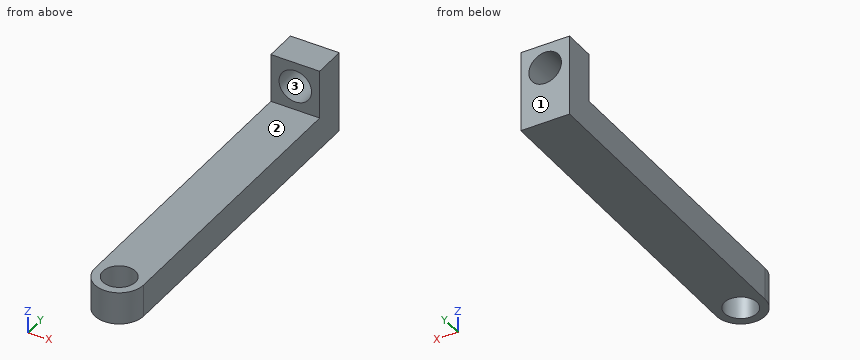
Autodesk Inventor part; units mm, degrees
ref_plane "YZ Plane" through (0, 0, 0) normal (1, 0, 0) x (0, 1, 0)
ref_plane "XZ Plane" through (0, 0, 0) normal (0, 1, 0) x (-1, 0, 0)
ref_plane "XY Plane" through (0, 0, 0) normal (0, 0, 1) x (1, 0, 0)
sketch "草圖1" plane through (0, 0, 0) normal (0, 0, 1) x (1, 0, 0)
  circle A0 centre (0, 0) radius 5
  line L0 (0, 0) -> (0, 100) construction
  line L1 (-7.5, 0) -> (-7.5, 100)
  line L2 (7.5, 100) -> (7.5, 0)
  arc A1 (-7.5, 0) -> (7.5, 0) centre (0, 0) ccw
  arc A2 (7.5, 100) -> (-7.5, 100) centre (0, 100) ccw
  line L3 (-7.5, 100) -> (7.5, 100)
  point P0 (0, 50)
  dimension "d0" = 10
  dimension "d1" = 15
  dimension "d2" = 100
extrude "擠出1" add sketch "草圖1" along normal blind 10 contours L1 L3 L2 A1
sketch "草圖2" plane through (-7.5, 100, 0) normal (0, 1, 0) x (1, 0, 0)
  line L0 (15, -10) -> (0, -10)
  line L1 (15, -25) -> (0, -25)
  line L2 (0, -25) -> (0, -10)
  line L3 (0, -10) -> (15, -10)
  line L4 (15, -10) -> (15, -25)
  line L5 (15, -25) -> (0, -10) construction
  line L6 (0, -25) -> (15, -10) construction
  line L7 (15, 0) -> (15, -10)
  circle A0 centre (7.5, -17.5) radius 5
  point P0 (7.5, 0)
  point P1 (15, -10)
  dimension "d13" = 0
  dimension "d14" = 15
  dimension "d15" = 10
extrude "擠出2" add sketch "草圖2" against normal blind 10
Input: part model. Units: mm. Frame: model coordinates. Face numbers are marked on the shaded views. Coordinates: 2 decimals unless noted, no trailing zeros. Loops run counter-clockwise (first coordinate to the right, second up) from the corner with the lowest first, then second, coordinate; pieces in that order, holes last. Notation, with made-up numbers: M -16.5,-40 L 24.5,-40 A11 cw 24.5,-33 Z; hole C 8.25,63.5 d7. An arc over 180 degrees is marked long. One line per item, written item: value.
(1) Section D-D (y = 33). Output: boundary loops of the cut face in (x, z), and give its area (3 significant figures).
Filled in:
outline: M -7.5,0 L 7.5,0 L 7.5,10 L -7.5,10 Z
area: 150 mm^2
(2) Pin query (flat end, axial travel): pin 1 (5 mm diameter, centred on x = -3, z = 14, fed in from +Y); pin 2 (1 mm diameter, centred on x = 5, z = 16, fed in from -Y); pin 3 (4 mm diameter, centred on x = 1.5, y = 36.5, fed in from +Z). Return the tip coordinate at first contact, or that it passes through.
Filled in:
pin 1: y = 100
pin 2: y = 90
pin 3: z = 10
(3) Section C-C (z = 3.5). Output: boundary loops of the cut face in (x, y), and give its area (3 significant figures).
Filled in:
outline: M -7.5,0 A7.5 ccw 7.5,0 L 7.5,100 L -7.5,100 Z; hole C 0,0 d10
area: 1,510 mm^2
(4) Section B-B (x = 0). Output: boundary loops of the cut face in (y, z).
Filled in:
outline: M -7.5,0 L -5,0 L -5,10 L -7.5,10 Z; M 5,0 L 100,0 L 100,12.5 L 90,12.5 L 90,10 L 5,10 Z; M 90,22.5 L 100,22.5 L 100,25 L 90,25 Z
(5) Section A-A (z = 17.5). Output: boundary loops of the cut face in (x, y), and give its area (3 significant figures).
Filled in:
outline: M -7.5,90 L -5,90 L -5,100 L -7.5,100 Z; M 5,90 L 7.5,90 L 7.5,100 L 5,100 Z
area: 50.0 mm^2
(6) Pull-direction query (Z, two-part tool) for the marked faces 1, 2 and 3; classes: +Z half, -Z half, draft (parallel to the pull), parting line (faces both ways), or undercut.
Filled in:
face 1: draft
face 2: +Z half
face 3: undercut
(7) Line query: line 1 along Y through (x, z) = (0, 5.25); line 2 along Z through (x, y) = (0, 92.75); line 3 along X through (y, z) = (95.75, 17.5). Output: solid intervals per line, ascending. Write a range as from..to.
Filled in:
line 1: -7.5..-5, 5..100
line 2: 0..12.5, 22.5..25
line 3: -7.5..-5, 5..7.5
